The model under review builds one solid part; all positions refer to its coordinate system, in mm. A direction names the side the tool comes from. Give positions to 0.01 mm unless a question says otherwise; leave off trailing zeros. Loops run counter-clockwise (first coordinate to the right, second up) from the corner with the lowest first, then second, coordinate; pieces in that order, holes last. Notation, with made-up numbers: M 37,66 L 66,66 A22 cw 66,83 Z; hole C 39.5,66 d4. An arc over 180 degrees is marked long. One line per item, written item: value. Start each with the question number.
Q1. To check wall thickness, follow line 1 along Y through (x, z) = (19.5, 8); line 2 along Y through (x, z) = (35, 14); line 3 along Z through (x, y) = (40, 0.5). State the ranges of each line that lie inside material, in increasing order. Write a range as from..to.
Q2. We need section B-B on z = 11. Write out the cut boundary in (x, y), plus the area to 3 significant figures.
Q3. Mouldability with a two-part tool opening along X and no side actions: class faces 1 (the face through (0, 1, 16)), 2 (the face through (58, 1, 16)), 3 (the face through (6, 7, 7.5)), 4 (the face through (50, 10, 4)) as released by +X, released by -X, zero draft, split by the parting line, or undercut.
Q4. For faces 5 (the face through (22, 3, 16)), 6 (the face through (54, 10, 4)), 7 (the face through (29, 2, 23)), list the 3-axis set-ups (+Z, -Z, +X, -X, +Y, -Y) from which the entire face can be reached by the end or side of a thin tool; tool diameter is ignored.
Q5. We need section A-A on z = 28.5. Write out the cut boundary in (x, y).
Q6. For pin 1 (2 mm diameter, centred on y = 7.5, z = 4.5, fed in from +X); pin 2 (3.5 mm diameter, centred on x = 5.5, y = 6, fed in from -Z); pin 3 (0.6 mm diameter, centred on x = 47.5, y = 1, fed in from +Z), all flat-tipped, find the tip position at first contact; note any pin that passes through.
```python
from build123d import *

# Parameters (mm, degrees)
SKETCH1_W           = 58
SKETCH1_H           = 32
EXTRUDE1_DEPTH      = 2
CUT_EXTRUDE1_REACH  = 4
SKETCH2_R           = 0.5
SKETCH3_W           = 5
SKETCH3_H           = 5
EXTRUDE2_DEPTH      = 8
SKETCH10_W          = 3
SKETCH10_H          = 3
FLASH_LED_BOX_DEPTH = 9
SKETCH12_W          = 3
SKETCH12_H          = 3
SKETCH12_W_2        = 2.4
SKETCH12_H_2        = 2.4
EXTRUDE4_DEPTH      = 1
SKETCH13_W          = 2.04
SKETCH13_H          = 1.64
EXTRUDE5_DEPTH      = 1
SKETCH14_W          = 24
SKETCH14_H          = 5
EXTRUDE6_DEPTH      = 5
EXTRUDE7_DEPTH      = 7
EXTRUDE8_DEPTH      = 6
SKETCH18_W          = 20
SKETCH18_H          = 5
TO_LCD_DEPTH        = 3
SKETCH19_W          = 14
SKETCH19_H          = 8
FLASH_MEMORY_DEPTH  = 2
SKETCH20_W          = 7
SKETCH20_H          = 3
EXTRUDE11_DEPTH     = 3
SKETCH21_R          = 3.5
EXTRUDE12_DEPTH     = 5
FILLET1_R           = 2


with BuildPart() as part:
    # Sketch1 → Extrude1 (new body)
    with BuildSketch(Plane(origin=(0, 0, 0), x_dir=(1, 0, 0), z_dir=(0, 1, 0))):
        with Locations((29, -16)):
            Rectangle(SKETCH1_W, SKETCH1_H)
    extrude(amount=EXTRUDE1_DEPTH)

    # Sketch2 → Cut-Extrude1 (cut, up to next)
    with BuildSketch(Plane(origin=(0, 2, 0), x_dir=(-1, 0, 0), z_dir=(0, 1, 0)), mode=Mode.PRIVATE) as cut_extrude1_sk1:
        with Locations((-55.557, 2.464)):
            Circle(SKETCH2_R)
    cut_extrude1_tool1 = extrude(cut_extrude1_sk1.sketch, amount=-CUT_EXTRUDE1_REACH, mode=Mode.PRIVATE) & part.part
    add(cut_extrude1_tool1.solids().sort_by_distance((55.557, 2, 2.464))[0], mode=Mode.SUBTRACT)
    # Sketch2 → Cut-Extrude1 (cut, up to next)
    with BuildSketch(Plane(origin=(0, 2, 0), x_dir=(-1, 0, 0), z_dir=(0, 1, 0)), mode=Mode.PRIVATE) as cut_extrude1_sk2:
        with Locations((-55.557, 9.535)):
            Circle(SKETCH2_R)
    cut_extrude1_tool2 = extrude(cut_extrude1_sk2.sketch, amount=-CUT_EXTRUDE1_REACH, mode=Mode.PRIVATE) & part.part
    add(cut_extrude1_tool2.solids().sort_by_distance((55.557, 2, 9.535))[0], mode=Mode.SUBTRACT)
    # Sketch2 → Cut-Extrude1 (cut, up to next)
    with BuildSketch(Plane(origin=(0, 2, 0), x_dir=(-1, 0, 0), z_dir=(0, 1, 0)), mode=Mode.PRIVATE) as cut_extrude1_sk3:
        with Locations((-55.557, 27)):
            Circle(SKETCH2_R)
    cut_extrude1_tool3 = extrude(cut_extrude1_sk3.sketch, amount=-CUT_EXTRUDE1_REACH, mode=Mode.PRIVATE) & part.part
    add(cut_extrude1_tool3.solids().sort_by_distance((55.557, 2, 27))[0], mode=Mode.SUBTRACT)
    # Sketch2 → Cut-Extrude1 (cut, up to next)
    with BuildSketch(Plane(origin=(0, 2, 0), x_dir=(-1, 0, 0), z_dir=(0, 1, 0)), mode=Mode.PRIVATE) as cut_extrude1_sk4:
        with Locations((-2.022, 27)):
            Circle(SKETCH2_R)
    cut_extrude1_tool4 = extrude(cut_extrude1_sk4.sketch, amount=-CUT_EXTRUDE1_REACH, mode=Mode.PRIVATE) & part.part
    add(cut_extrude1_tool4.solids().sort_by_distance((2.022, 2, 27))[0], mode=Mode.SUBTRACT)
    # Sketch2 → Cut-Extrude1 (cut, up to next)
    with BuildSketch(Plane(origin=(0, 2, 0), x_dir=(-1, 0, 0), z_dir=(0, 1, 0)), mode=Mode.PRIVATE) as cut_extrude1_sk5:
        with Locations((-2.022, 2.464)):
            Circle(SKETCH2_R)
    cut_extrude1_tool5 = extrude(cut_extrude1_sk5.sketch, amount=-CUT_EXTRUDE1_REACH, mode=Mode.PRIVATE) & part.part
    add(cut_extrude1_tool5.solids().sort_by_distance((2.022, 2, 2.464))[0], mode=Mode.SUBTRACT)

    # Sketch3 → Extrude2 (add)
    with BuildSketch(Plane(origin=(0, 2, 0), x_dir=(-1, 0, 0), z_dir=(0, 1, 0))):
        with Locations((-52.021432188, 5.9995)):
            Rectangle(SKETCH3_W, SKETCH3_H)
    extrude(amount=EXTRUDE2_DEPTH)

    # Sketch6 → Revolve1 (revolve)
    with BuildSketch(Plane(origin=(52.021432188, 0, 0), x_dir=(0, 0, -1), z_dir=(1, 0, 0))):
        with BuildLine():
            Line((-3.4995, 10), (-5.9995, 10))
            Line((-5.9995, 10), (-5.9995, 11.443375673))
            ThreePointArc((-5.9995, 11.443375673), (-4.556124327, 11.056624327), (-3.4995, 10))
        make_face()
    revolve(axis=Axis((52.021432188, 11.443375673, 5.9995), (0, -1, 0)))

    # Sketch10 → flash led box (add)
    with BuildSketch(Plane(origin=(0, 2, 0), x_dir=(-1, 0, 0), z_dir=(0, 1, 0))):
        with Locations((-6.022, 6)):
            Rectangle(SKETCH10_W, SKETCH10_H)
    extrude(amount=FLASH_LED_BOX_DEPTH)

    # Sketch12 → Extrude4 (add)
    with BuildSketch(Plane(origin=(0, 11, 0), x_dir=(-1, 0, 0), z_dir=(0, 1, 0))):
        with Locations((-6.022, 6)):
            Rectangle(SKETCH12_W, SKETCH12_H)
        with Locations((-6.022, 6)):
            Rectangle(SKETCH12_W_2, SKETCH12_H_2, mode=Mode.SUBTRACT)
    extrude(amount=EXTRUDE4_DEPTH)

    # Sketch13 → Extrude5 (add)
    with BuildSketch(Plane(origin=(0, 11, 0), x_dir=(-1, 0, 0), z_dir=(0, 1, 0))):
        with Locations((-6.022, 6)):
            Rectangle(SKETCH13_W, SKETCH13_H)
    extrude(amount=EXTRUDE5_DEPTH)

    # Sketch14 → Extrude6 (add)
    with BuildSketch(Plane(origin=(0, 2, 0), x_dir=(-1, 0, 0), z_dir=(0, 1, 0))):
        with Locations((-29, 29.5)):
            Rectangle(SKETCH14_W, SKETCH14_H)
    extrude(amount=EXTRUDE6_DEPTH)

    # Sketch16 → Extrude7 (add)
    with BuildSketch(Plane.XY.offset(32)):
        with BuildLine():
            Line((18, 7), (40, 7))
            ThreePointArc((40, 7), (40.707106781, 6.707106781), (41, 6))
            Line((41, 6), (41, 1))
            ThreePointArc((41, 1), (40.707106781, 0.292893219), (40, 0))
            Line((40, 0), (18, 0))
            ThreePointArc((18, 0), (17.292893219, 0.292893219), (17, 1))
            Line((17, 1), (17, 6))
            ThreePointArc((17, 6), (17.292893219, 6.707106781), (18, 7))
        make_face()
    extrude(amount=EXTRUDE7_DEPTH)

    # Sketch17 → Extrude8 (add)
    with BuildSketch(Plane.XY.offset(39)):
        with BuildLine():
            Line((18.5, 4.5), (39.5, 4.5))
            ThreePointArc((39.5, 4.5), (39.853553391, 4.353553391), (40, 4))
            Line((40, 4), (40, 3))
            ThreePointArc((40, 3), (39.853553391, 2.646446609), (39.5, 2.5))
            Line((39.5, 2.5), (18.5, 2.5))
            ThreePointArc((18.5, 2.5), (18.146446609, 2.646446609), (18, 3))
            Line((18, 3), (18, 4))
            ThreePointArc((18, 4), (18.146446609, 4.353553391), (18.5, 4.5))
        make_face()
    extrude(amount=EXTRUDE8_DEPTH)

    # Sketch18 → to lcd (add)
    with BuildSketch(Plane(origin=(0, 2, 0), x_dir=(-1, 0, 0), z_dir=(0, 1, 0))):
        with Locations((-29, 2.5)):
            Rectangle(SKETCH18_W, SKETCH18_H)
    extrude(amount=TO_LCD_DEPTH)

    # Sketch19 → flash memory (add)
    with BuildSketch(Plane(origin=(0, 2, 0), x_dir=(-1, 0, 0), z_dir=(0, 1, 0))):
        with Locations((-29, 16)):
            Rectangle(SKETCH19_W, SKETCH19_H)
    extrude(amount=FLASH_MEMORY_DEPTH)

    # Sketch20 → Extrude11 (add)
    with BuildSketch(Plane(origin=(0, 2, 0), x_dir=(-1, 0, 0), z_dir=(0, 1, 0))):
        with Locations((-8.02, 1.5)):
            Rectangle(SKETCH20_W, SKETCH20_H)
    extrude(amount=EXTRUDE11_DEPTH)

    # Sketch21 → Extrude12 (add)
    with BuildSketch(Plane(origin=(0, 0, 0), x_dir=(-1, 0, 0), z_dir=(0, 0, -1))):
        with Locations((-8.02, 1)):
            Circle(SKETCH21_R)
    extrude(amount=EXTRUDE12_DEPTH)

    # Fillet1
    fillet1_edges = [part.edges().sort_by_distance(p)[0] for p in [
        (11.52, 1, -5),
    ]]
    fillet(fillet1_edges, radius=FILLET1_R)


solid = part.part
```
Solved:
1. line 1: 0..2
1. line 2: 0..4
1. line 3: 0..39
2. outline: M 0,0 L 58,0 L 58,2 L 0,2 Z
2. area: 116 mm2
3. face 1: released by -X
3. face 2: released by +X
3. face 3: zero draft
3. face 4: undercut
4. face 5: -X, +Y
4. face 6: -Z, +X, +Y
4. face 7: +Y
5. outline: M 0,0 L 58,0 L 58,2 L 41,2 L 41,7 L 17,7 L 17,2 L 0,2 Z
6. pin 1: x = 54.52
6. pin 2: z = 0
6. pin 3: z = 32
